from build123d import *

# Parameters (mm, degrees)
SALIENTE_EXTRUIR1_DEPTH = 30
CROQUIS2_W              = 30
CROQUIS2_H              = 30
SALIENTE_EXTRUIR3_DEPTH = 150


with BuildPart() as part:
    # Croquis1 → Saliente-Extruir1 (new body)
    with BuildSketch(Plane.XY):
        Polygon((-130, 135), (-130, -15), (-100, -15), (-100, 105), (20, 105), (20, 135), align=None)
    extrude(amount=SALIENTE_EXTRUIR1_DEPTH)

    # Croquis2 → Saliente-Extruir3 (add)
    with BuildSketch(Plane.XY):
        with Locations((-115, 0)):
            Rectangle(CROQUIS2_W, CROQUIS2_H)
    extrude(amount=SALIENTE_EXTRUIR3_DEPTH)


solid = part.part
The model under review builds one solid part; all positions refer to its coordinate system, in mm. A direction names the side the tool comes from. Round coordinates to 2 decimals unless told otherwise and drop trailing zeros. Loops run counter-clockwise (first coordinate to the right, second up) from the corner with the lowest first, then second, coordinate; pieces in that order, holes last. Notation, with made-up numbers: M 9,46.25 L 55,46.25 A19 cw 55,73.25 Z; hole C -7,36 d8. An arc over 180 degrees is marked long. Answer as CSV lines item,"result".
1. We need section D-D (z = 136). Give the boundary of the cut face in (x, y).
Outcome:
outline,"M -130,-15 L -100,-15 L -100,15 L -130,15 Z"
2. We need section B-B (x = -117.5). Give the boundary of the cut face in (y, z).
Outcome:
outline,"M -15,0 L 135,0 L 135,30 L 15,30 L 15,150 L -15,150 Z"
3. Insertion check: pin 1 Ø15 at (x, z) = (-59.5, 14) entering from -Y; pin 2 Ø9 at (x, z) = (-122, 83) entering from +Y. Each pin has a flat end and moves straight along its axis. Give the tip position at first contact, or say it passes through.
Outcome:
pin 1,"stops at y = 105"
pin 2,"stops at y = 15"
4. Draft analysis for pull direction Z (two halves, no side actions). For faces 4 (the face through (-89, 111, 0)), 5 (the face through (-89, 116, 30)), 6 (the face through (-115, -15, 74)), state which applies: pulls with the +Z half, pulls with the -Z half, needs draft (parallel to the pull), parting line crosses it, or undercut.
Outcome:
face 4,"pulls with the -Z half"
face 5,"pulls with the +Z half"
face 6,"needs draft"
5. For faces 1 (the face through (-115, 15, 89)), 2 (the face through (-100, 4, 41)), 3 (the face through (-54, 135, 15)), list the 3-axis set-ups (+Z, -Z, +X, -X, +Y, -Y) from which the entire face can be reached by the end or side of a thin tool; tool diameter is ignored.
Outcome:
face 1,"+Z, +X, -X, +Y"
face 2,"+Z, -Z, +X, -Y"
face 3,"+Z, -Z, +X, -X, +Y"
6. We need section A-A (z = 21). Give the boundary of the cut face in (x, y).
Outcome:
outline,"M -130,-15 L -100,-15 L -100,105 L 20,105 L 20,135 L -130,135 Z"
7. To check wall thickness, follow L1, parallel to X at y = -6.5, z = 134.5; L2, parallel to Z at x = -113, y = 125.5; L3, parallel to Y at x = 9.5, z = 15. State the ranges of each line that lie inside material, in increasing order. Write a range as [from, to].
Outcome:
L1,"x = [-130, -100]"
L2,"z = [0, 30]"
L3,"y = [105, 135]"
8. We need section C-C (y = 114.5). Give the boundary of the cut face in (x, z).
Outcome:
outline,"M -130,0 L 20,0 L 20,30 L -130,30 Z"
